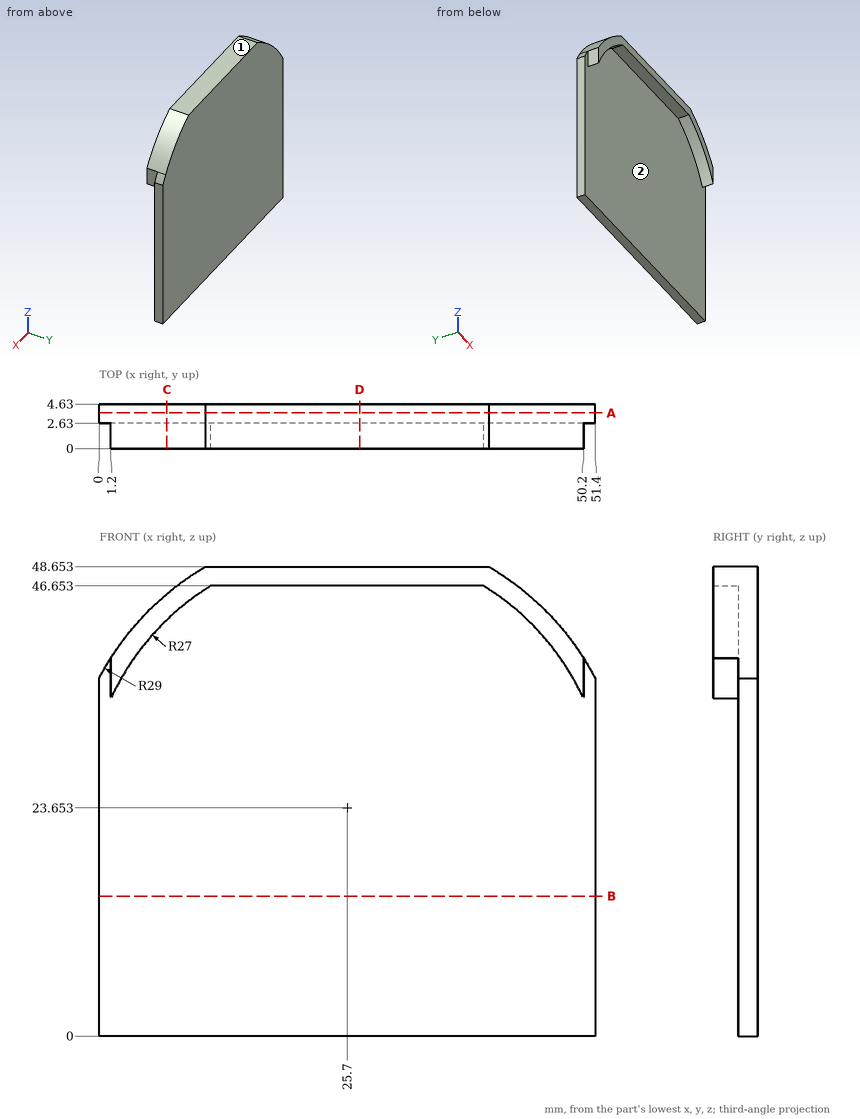
Job drawing, mm, ordinate dimensions from the low corner. One solid piece. Coordinates: 2 decimals unless noted, no trailing zeros. Order: outer loops, then holes, each group sorted by start corner. A loop starts at its lowest first (then second) coordinate and runs counter-clockwise, first axis right, second up. Notation, with made-up numbers: M 7,-28.5 L 46,-28.5 A12 ccw 46,-13.5 Z; hole C -25.75,-32 d5. An arc over 180 degrees is marked long. Return JSON: item names as keys, results as strings.
1. Pull direction X, two halves, no side cores. Call the marked faces 1 and 2: +X half, -X half, draft (parallel to the pull), parting line (faces both ways), or undercut.
Ans:
{"face 1": "draft", "face 2": "undercut"}
2. Saw through at D-D (x = 27). Give the cut face in (y, z), and give its area (3 significant figures).
Ans:
{"outline": "M 0,46.65 L 2.63,46.65 L 2.63,0 L 4.63,0 L 4.63,48.65 L 0,48.65 Z", "area": "103 mm^2"}
3. Saw through at A-A (y = 3.7). Give the cut face in (x, z).
Ans:
{"outline": "M 0,0 L 51.4,0 L 51.4,37.09 A29 ccw 40.4,48.65 L 11,48.65 A29 ccw 0,37.09 Z"}
4. Saw through at B-B (z = 14.5). Give the cut face in (x, y), and give its area (3 significant figures).
Ans:
{"outline": "M 0,2.63 L 51.4,2.63 L 51.4,4.63 L 0,4.63 Z", "area": "103 mm^2"}
5. Drill centre lines: probe 1 along Y at (x, z) = (35, 5.5); probe 2 along X at (y, z) = (0.25, 43); probe 3 along Z at (x, y) = (15.5, 0.45). Where is each one in solid material? Low to high.
Ans:
{"probe 1": "2.63 to 4.63", "probe 2": "4.1 to 6.87, 44.53 to 47.3", "probe 3": "46.65 to 48.65"}
6. Saw through at C-C (x = 7). Give the cut face in (y, z).
Ans:
{"outline": "M 0,43.13 L 2.63,43.13 L 2.63,0 L 4.63,0 L 4.63,45.82 L 0,45.82 Z"}
7. Flat gauge pins, fed straight in: pin 1 (0.8 mm diameter, centred on y = 1.5, z = 37, fed in from -X); pin 2 (0.8 mm diameter, centred on x = 32.5, y = 1.5, fed in from -Z). Where does each tip first touch, or does it go through?
Ans:
{"pin 1": "x = 1.2", "pin 2": "z = 46.65"}
